The drawing under review shows one solid part. Ordinate dimensions are in mm from its lowest x, y, z. A direction names the side the tool comes from. Round coordinates to 2 decimals unless told otherwise and drop trailing zeros. Write each loop counter-clockwise with the first axis right and the second up, starting at its lowest first coordinate (ties: lowest second). Pieces come first, ordered by that corner, then holes. Notation, with made-up numbers: (-3.5, 14.25) -> (24.5, 14.25) arc R23 ccw to (24.5, 39.25) -> close; hole circle Ø6 at (38, 33). An arc over 180 degrees is marked (long way). Answer in a Markdown table with one row per item.
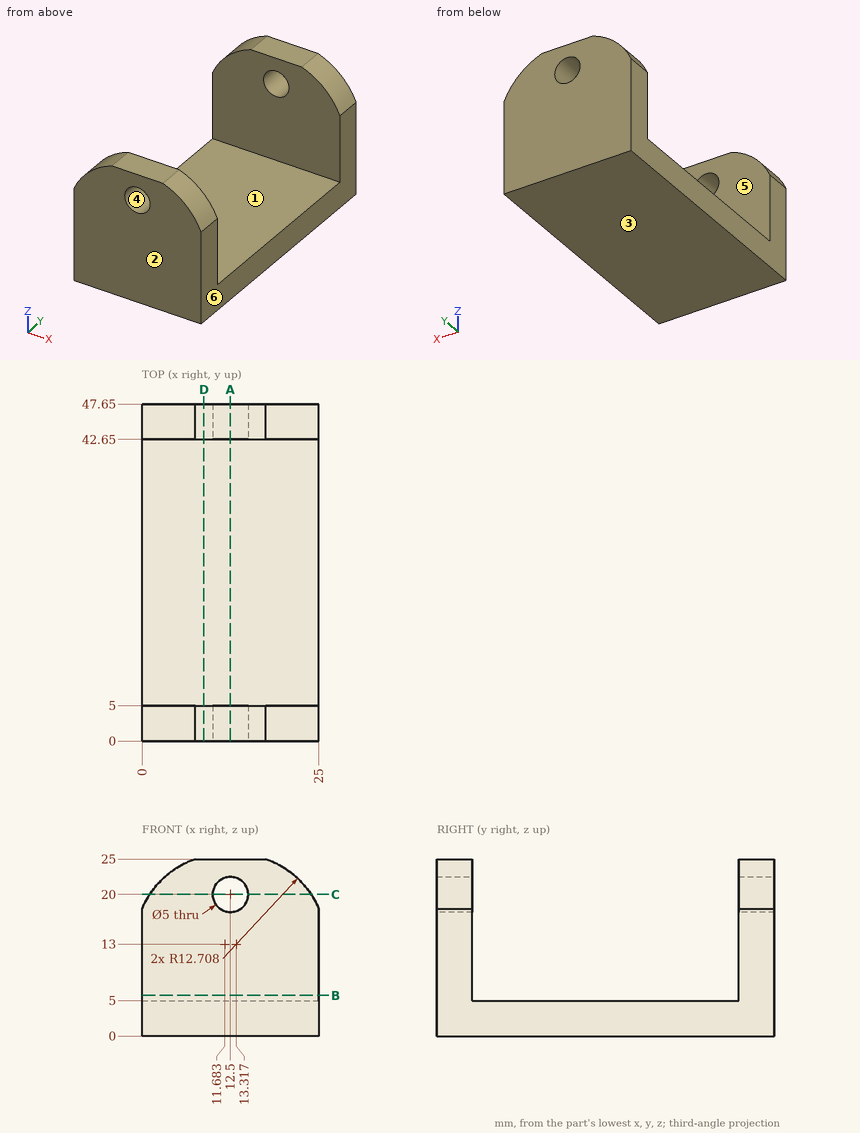
1) Mouldability with a two-part tool opening along Z and no side actions: class the marked faces 1, 2, 3 and 4 as pulls with the +Z half, pulls with the -Z half, needs draft (parallel to the pull), parting line crosses it, or undercut.
Solved:
| item | result |
|---|---|
| face 1 | pulls with the +Z half |
| face 2 | needs draft |
| face 3 | pulls with the -Z half |
| face 4 | undercut |
2) Clearance check with a flat-ended pin moving along its axis: pin 1 Ø3 at (x, y) = (7, 26.5) entering from -Z. State where the tip first meets the part, or that it passes through.
Solved:
| item | result |
|---|---|
| pin 1 | z = 0 |
3) For line 1 (Y direction, x = 9.75, z = 15.75); line 2 (Z direction, x = 4, y = 31); line 3 (X direction, y = 3.6, z = 20), list the stretches that pass through material, from the lowest coordinate up. Write a range as [from, to].
Solved:
| item | result |
|---|---|
| line 1 | [0, 5], [42.65, 47.65] |
| line 2 | [0, 5] |
| line 3 | [1.08, 10], [15, 23.92] |
4) For the marked faces 5 and 6, list the 3-axis set-ups (+Z, -Z, +X, -X, +Y, -Y) from which the entire face can be reached by the end or side of a thin tool; tool diameter is ignored.
Solved:
| item | result |
|---|---|
| face 5 | +Z, +X, -X |
| face 6 | +Z, -Z, +X, +Y, -Y |
5) Consider section A-A on x = 12.5. State the section outline as (y, z) points, then the cut area to 3 significant figures.
Solved:
| item | result |
|---|---|
| outline | (0, 0) -> (47.65, 0) -> (47.65, 17.5) -> (42.65, 17.5) -> (42.65, 5) -> (5, 5) -> (5, 17.5) -> (0, 17.5) -> close; (0, 22.5) -> (5, 22.5) -> (5, 25) -> (0, 25) -> close; (42.65, 22.5) -> (47.65, 22.5) -> (47.65, 25) -> (42.65, 25) -> close |
| area | 388 mm² |
6) Consider section D-D on x = 8.75. State the section outline as (y, z) points, then the cut area to 3 significant figures.
Solved:
| item | result |
|---|---|
| outline | (0, 0) -> (47.65, 0) -> (47.65, 25) -> (42.65, 25) -> (42.65, 5) -> (5, 5) -> (5, 25) -> (0, 25) -> close |
| area | 438 mm² |
7) Consider section B-B on z = 5.75. State the section outline as (x, y) points.
Solved:
| item | result |
|---|---|
| outline | (0, 0) -> (25, 0) -> (25, 5) -> (0, 5) -> close; (0, 42.65) -> (25, 42.65) -> (25, 47.65) -> (0, 47.65) -> close |
8) Consider section C-C on z = 20. State the section outline as (x, y) points.
Solved:
| item | result |
|---|---|
| outline | (1.08, 0) -> (10, 0) -> (10, 5) -> (1.08, 5) -> close; (1.08, 42.65) -> (10, 42.65) -> (10, 47.65) -> (1.08, 47.65) -> close; (15, 0) -> (23.92, 0) -> (23.92, 5) -> (15, 5) -> close; (15, 42.65) -> (23.92, 42.65) -> (23.92, 47.65) -> (15, 47.65) -> close |
